Verification items for the finished model (mm, model axes). Face numbers are marked on the shaded views. Round coordinates to 2 decimals unless told otherwise and drop trailing zeros. Write each loop counter-clockwise with the first axis right and the second up, starting at its lowest first coordinate (ties: lowest second). Pieces come first, ordered by that corner, then holes. Notation, with made-up numbers: (4, -6.5) - (21, -6.5) arc R9 cw to (21, 7.5) - close; hole circle Ø4 at (80, 47.5). An arc over 180 degrees is marked (long way). Answer as a JSON object with one key per item and string values. Group by question number.
1) Section check A-A (z = 0). Enter the section's corners in (x, y).
2) Go/stop test with flat-tipped pins: pin 1 Ø6 at (x, z) = (49, 9) entering from -Y; pin 2 Ø10 at (x, z) = (14, -35) entering from +Y. Record where each tip stops, or that it passes through.
3) Section check D-D (z = -35). Enter the section's corners in (x, y).
4) Section check B-B (x = -30.8). Enter the section's corners in (y, z).
5) Thickness scan on line 1 (X direction, y = 3.55, z = -31.5); line 2 (Z direction, x = -15.5, y = 5.75); line 3 (Z direction, x = -30.8, y = 1.2). Record the ranges inside material, lowest first.
6) Mould release check, pull along X, two halves, no side actions. Record for the marked faces 1 and 2: +X half, -X half, draft (parallel to the pull), parting line (faces both ways), or undercut.
7) Section check C-C (y = 4.45). Enter the section's corners in (x, z).
```python
from build123d import *

# Parameters (mm, degrees)
SKETCH1_W                                       = 133
SKETCH1_H                                       = 91
BOSS_EXTRUDE1_DEPTH                             = 6
SKETCH2_W                                       = 127
SKETCH2_H                                       = 85
CUT_EXTRUDE1_DEPTH                              = 3
FILLET1_R                                       = 2.5
CSK_FOR_M3_FLAT_HEAD_MACHINE_SCREW1_D           = 3.4
CSK_FOR_M3_FLAT_HEAD_MACHINE_SCREW1_DEPTH       = 17.38
CSK_FOR_M3_FLAT_HEAD_MACHINE_SCREW1_CSINK_D     = 6.3
CSK_FOR_M3_FLAT_HEAD_MACHINE_SCREW1_CSINK_ANGLE = 90
CSK_FOR_M3_FLAT_HEAD_MACHINE_SCREW1_TIP         = 1.021463052


with BuildPart() as part:
    # Sketch1 → Boss-Extrude1 (new body)
    with BuildSketch(Plane(origin=(0, 0, 0), x_dir=(1, 0, 0), z_dir=(0, 1, 0))):
        Rectangle(SKETCH1_W, SKETCH1_H)
    extrude(amount=BOSS_EXTRUDE1_DEPTH)

    # Sketch2 → Cut-Extrude1 (cut)
    with BuildSketch(Plane(origin=(0, 6, 0), x_dir=(1, 0, 0), z_dir=(0, 1, 0))):
        Rectangle(SKETCH2_W, SKETCH2_H)
    extrude(amount=-CUT_EXTRUDE1_DEPTH, mode=Mode.SUBTRACT)

    # Fillet1
    fillet1_edges = [part.edges().sort_by_distance(p)[0] for p in [
        (63.5, 4.5, -42.5),
        (63.5, 4.5, 42.5),
        (-63.5, 4.5, 42.5),
        (-63.5, 4.5, -42.5),
        (66.5, 3, 45.5),
        (-66.5, 3, 45.5),
        (-66.5, 3, -45.5),
        (66.5, 3, -45.5),
    ]]
    fillet(fillet1_edges, radius=FILLET1_R)

    # CSK for M3 Flat Head Machine Screw1
    with Locations(Plane(origin=(0, 3, 0), x_dir=(1, 0, 0), z_dir=(0, 1, 0))):
        with Locations((-30.8, 0), (30.8, 0)):
            CounterSinkHole(CSK_FOR_M3_FLAT_HEAD_MACHINE_SCREW1_D / 2, CSK_FOR_M3_FLAT_HEAD_MACHINE_SCREW1_CSINK_D / 2, depth=CSK_FOR_M3_FLAT_HEAD_MACHINE_SCREW1_DEPTH, counter_sink_angle=CSK_FOR_M3_FLAT_HEAD_MACHINE_SCREW1_CSINK_ANGLE)
            with Locations((0, 0, -(CSK_FOR_M3_FLAT_HEAD_MACHINE_SCREW1_DEPTH + CSK_FOR_M3_FLAT_HEAD_MACHINE_SCREW1_TIP / 2))):  # 118° drill point
                Cone(0, CSK_FOR_M3_FLAT_HEAD_MACHINE_SCREW1_D / 2, CSK_FOR_M3_FLAT_HEAD_MACHINE_SCREW1_TIP, mode=Mode.SUBTRACT)


solid = part.part
```
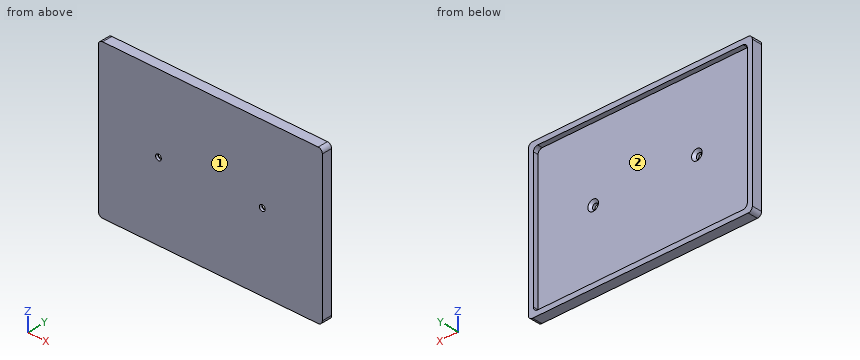
Returned:
{
 "1": {"outline": "(-66.5, 0) - (-32.5, 0) - (-32.5, 1.55) - (-33.95, 3) - (-63.5, 3) - (-63.5, 6) - (-66.5, 6) - close; (-29.1, 0) - (29.1, 0) - (29.1, 1.55) - (27.65, 3) - (-27.65, 3) - (-29.1, 1.55) - close; (32.5, 0) - (66.5, 0) - (66.5, 6) - (63.5, 6) - (63.5, 3) - (33.95, 3) - (32.5, 1.55) - close"},
 "2": {"pin 1": "y = 0", "pin 2": "y = 3"},
 "3": {"outline": "(-66.5, 0) - (66.5, 0) - (66.5, 6) - (63.5, 6) - (63.5, 3) - (-63.5, 3) - (-63.5, 6) - (-66.5, 6) - close"},
 "4": {"outline": "(0, -45.5) - (6, -45.5) - (6, -42.5) - (3, -42.5) - (3, -3.15) - (1.55, -1.7) - (0, -1.7) - close; (0, 1.7) - (1.55, 1.7) - (3, 3.15) - (3, 42.5) - (6, 42.5) - (6, 45.5) - (0, 45.5) - close"},
 "5": {"line 1": "-66.5 to -63.5, 63.5 to 66.5", "line 2": "-45.5 to -42.5, 42.5 to 45.5", "line 3": "-45.5 to -1.7, 1.7 to 45.5"},
 "6": {"face 1": "draft", "face 2": "undercut"},
 "7": {"outline": "(-66.5, -43) arc R2.5 ccw to (-64, -45.5) - (64, -45.5) arc R2.5 ccw to (66.5, -43) - (66.5, 43) arc R2.5 ccw to (64, 45.5) - (-64, 45.5) arc R2.5 ccw to (-66.5, 43) - close; hole (-63.5, -40) arc R2.5 ccw to (-61, -42.5) - (61, -42.5) arc R2.5 ccw to (63.5, -40) - (63.5, 40) arc R2.5 ccw to (61, 42.5) - (-61, 42.5) arc R2.5 ccw to (-63.5, 40) - close"}
}
